Can you work these out from the model? Positions are in its coordinate system, mm. A direction names the side the tool comes from. Coordinates: 2 decimals unless noted, no trailing zeros. Order: outer loops, then holes, each group sorted by start corner. A loop starts at its lowest first (then second) coordinate and runs counter-clockwise, first axis right, second up. Notation, with made-up numbers: (9.5, 70.25) -> (63.5, 70.25) arc R26 cw to (63.5, 92.25) -> close; hole circle Ø1 at (-37, 72). An arc over 180 degrees is marked (long way). Answer in a Markdown table with one row per item. Add a question column.
1. If I drill on line 1 along Y through (x, z) = (11.75, 3); line 2 along X through (y, z) = (13.5, 8.75), over which ranges is the centre line in solid material (lowest first)? Write a range as [from, to].
2. Will these pins go through, and if not, where does the flat tip stop? pin 1 (5 mm diameter, centred on y = 7, z = 20, fed in from +X); pin 2 (3 mm diameter, centred on y = 15, z = 10.5, fed in from -X); pin 3 (6 mm diameter, centred on x = 18.5, y = 14, fed in from +Z).
3. Imagine slicing it at A-A on z = 7. Write out the boundary of the cut face in (x, y).
4. Imagine slicing it at B-B on y = 9. Write out the boundary of the cut face in (x, z).
5. On a 3-axis mill with a long thin cutter (end or side, diameter ignored), from which of +Z, -Z, +X, -X, +Y, -Y can I reach the whole of each face in a straight line? I mean faces 1 (the face through (10, 5, 20)), 2 (the face through (8, 10, 11)), 3 (the face through (25, 20, 5)). Say none if no direction works.
6. Imagine slicing it at C-C on x = 15. Write out the boundary of the cut face in (y, z).
from build123d import *

# Parameters (mm, degrees)
F0_W     = 10
F0_H     = 10
F1_DEPTH = 30
F2_W     = 10
F2_H     = 10
F3_DEPTH = 20
F4_W     = 10
F4_H     = 10
F5_DEPTH = 10


with BuildPart() as f1:
    # F0 (on Top) → F1 (new body)
    with BuildSketch(Plane.XY):
        with Locations((5, 5)):
            Rectangle(F0_W, F0_H)
    extrude(amount=F1_DEPTH)

    # F2 (on face) → F3 (join)
    with BuildSketch(Plane.YZ.offset(10)):
        with Locations((5, 5)):
            Rectangle(F2_W, F2_H)
    extrude(amount=F3_DEPTH)

    # F4 (on face) → F5 (join)
    with BuildSketch(Plane(origin=(0, 10, 0), x_dir=(-1, 0, 0), z_dir=(0, 1, 0))):
        with Locations((-25, 5)):
            Rectangle(F4_W, F4_H)
    extrude(amount=F5_DEPTH)


solid = f1.part
Answers follow:
| question | item | result |
|---|---|---|
| 1 | line 1 | y = [0, 10] |
| 1 | line 2 | x = [20, 30] |
| 2 | pin 1 | stops at x = 10 |
| 2 | pin 2 | stops at x = 20 |
| 2 | pin 3 | stops at z = 10 |
| 3 | outline | (0, 0) -> (30, 0) -> (30, 20) -> (20, 20) -> (20, 10) -> (0, 10) -> close |
| 4 | outline | (0, 0) -> (30, 0) -> (30, 10) -> (10, 10) -> (10, 30) -> (0, 30) -> close |
| 5 | face 1 | +Z, +X, +Y, -Y |
| 5 | face 2 | +Z, -Z, -X, +Y |
| 5 | face 3 | +Z, -Z, +X, -X, +Y |
| 6 | outline | (0, 0) -> (10, 0) -> (10, 10) -> (0, 10) -> close |
